Can you work these out from the model? Positions are in its coordinate system, mm. Face numbers are marked on the shaded views. A direction names the side the tool comes from. Give positions to 0.01 mm unless a question says otherwise; leave off trailing zeros. Loops run counter-clockwise (first coordinate to the right, second up) from the corner with the lowest first, then second, coordinate; pieces in that order, holes last. Notation, with made-up numbers: (-20, -38.5) - (8, -38.5) arc R6 ccw to (8, -30.5) - close; hole circle Ø6 at (79, -5.5). An arc over 180 degrees is marked (long way). Answer as a JSON object with one key per item and string values. Group by question number.
Item 1: Suppose I cut it at B-B on z = 10.25. Write out the boundary of the cut face in (x, y), and give its area (3 significant figures).
Item 2: Please list where these lines run through material, in increasing order: L1, parallel to Y at x = 7.75, z = 4.25; L2, parallel to X at y = 12.25, z = 8.25; L3, parallel to Y at x = 2, z = 1.25.
Item 3: Which directions (+Z, -Z, +X, -X, +Y, -Y) give clear straight access to the entire face, cutting with the end or side of a thin tool? Please do the marked faces 1, 2, 3, 4 and 5.
Item 4: Suppose I cut it at C-C on y = 14.5. Write out the boundary of the cut face in (x, z), and give its area (3 significant figures).
Item 5: Thinking about a two-plate mould opening in Y: for the marked faces 6, 7, 8 and 9, which applies, pulls with the +Y half, pulls with the -Y half, needs draft (parallel to the pull), parting line crosses it, or undercut?
Item 6: Will these pins go through, and if not, where does the flat tip stop? pin 1 (5 mm diameter, centred on x = 1.5, z = 6, fed in from -Y); pin 2 (3 mm diameter, centred on y = 10, z = 7, fed in from -X) (3 decimals); pin 3 (6 mm diameter, centred on x = 1, z = 3.5, fed in from -Y).
Item 7: Suppose I cut it at D-D on x = -9.5. Write out the boundary of the cut face in (y, z).
Item 8: Suppose I cut it at A-A on z = 4.25. Write out the boundary of the cut face in (x, y).
from build123d import *

# Parameters (mm, degrees)
F1_DEPTH = 12
F3_DEPTH = 10.5
F4_R     = 3
F5_R     = 1.35
F6_DEPTH = 8


with BuildPart() as f1:
    # F0 (on Top) → F1 (new body)
    with BuildSketch(Plane.XY):
        Polygon((-7.96441, 20), (-7.96441, 0), (-3.56441, 0), (-3.56441, 15.6), (12.03559, 15.6), (12.03559, 20), align=None)
    extrude(amount=F1_DEPTH)

    # F2 (on face) → F3 (cut)
    with BuildSketch(Plane.XY.offset(12)):
        Polygon((-6.66441, 0), (-5.76441, 0), (-5.76441, 17.8), (12.03559, 17.8), (12.03559, 18.7), (-6.66441, 18.7), align=None)
        Polygon((-5.76441, 17.8), (-5.76441, 0), (-4.76441, 0), (-4.76441, 16.8), (12.03559, 16.8), (12.03559, 17.8), align=None)
    extrude(amount=-F3_DEPTH, mode=Mode.SUBTRACT)

    # F4
    f4_edges = [f1.edges().sort_by_distance(p)[0] for p in [
        (-4.76441, 16.8, 6.75),
        (-3.56441, 15.6, 6),
    ]]
    fillet(f4_edges, radius=F4_R)

    # F5 (on Top) → F6 (join)
    with BuildSketch(Plane.XY):
        with BuildLine():
            ThreePointArc((-7.96441, 20), (-9.434479, 18.498851), (-11.331965, 17.59658))
            ThreePointArc((-11.331965, 17.59658), (-9.376537, 17.445554), (-7.96441, 16.084523))
            Line((-7.96441, 16.084523), (-7.96441, 20))
        make_face()
        with BuildLine():
            ThreePointArc((-7.96441, 13.515477), (-9.376537, 12.154446), (-11.331965, 12.00342))
            ThreePointArc((-11.331965, 12.00342), (-9.434479, 11.101149), (-7.96441, 9.6))
            Line((-7.96441, 9.6), (-7.96441, 13.515477))
        make_face()
        with BuildLine():
            ThreePointArc((-7.96441, 16.084523), (-9.376537, 17.445554), (-11.331965, 17.59658))
            ThreePointArc((-11.331965, 17.59658), (-13.46441, 14.8), (-11.331965, 12.00342))
            ThreePointArc((-11.331965, 12.00342), (-9.376537, 12.154446), (-7.96441, 13.515477))
            Line((-7.96441, 13.515477), (-7.96441, 16.084523))
        make_face()
        with Locations((-10.56441, 14.8)):
            Circle(F5_R, mode=Mode.SUBTRACT)
    extrude(amount=F6_DEPTH)


solid = f1.part
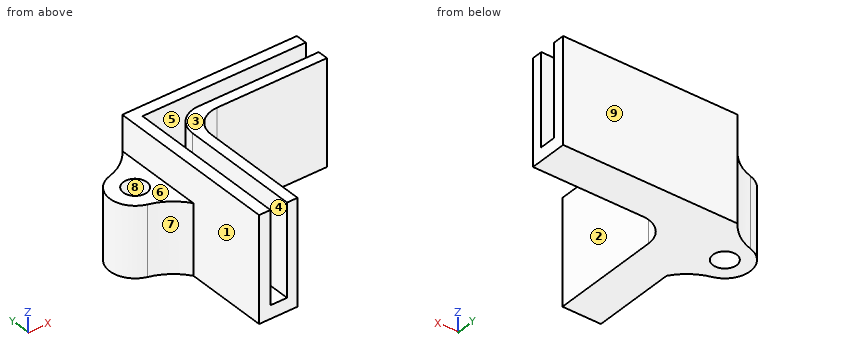
Worked out:
{
 "1": {"outline": "(-7.96, 0) - (-6.66, 0) - (-6.66, 18.7) - (12.04, 18.7) - (12.04, 20) - (-7.96, 20) - close; (-4.76, 0) - (-3.56, 0) - (-3.56, 12.6) arc R3 cw to (-0.56, 15.6) - (12.04, 15.6) - (12.04, 16.8) - (-1.76, 16.8) arc R3 ccw to (-4.76, 13.8) - close", "area": "89.2 mm2"},
 "2": {"L1": "y = 15.6 to 16.8, 18.7 to 20", "L2": "x = -7.96 to -6.66, -4.76 to -3.56", "L3": "y = 15.6 to 20"},
 "3": {"face 1": "+Z, -X, -Y", "face 2": "+Z, -Z, +X, -Y", "face 3": "+Z, +X, -X, +Y, -Y", "face 4": "+Z, -Y", "face 5": "+Z, +X"},
 "4": {"outline": "(-13.45, 0) - (-11.88, 0) - (-11.88, 8) - (-13.45, 8) - close; (-9.25, 0) - (-2.89, 0) - (-2.89, 12) - (-4.68, 12) - (-4.68, 1.5) - (-6.66, 1.5) - (-6.66, 12) - (-7.96, 12) - (-7.96, 8) - (-9.25, 8) - close", "area": "62.9 mm2"},
 "5": {"face 6": "needs draft", "face 7": "pulls with the -Y half", "face 8": "undercut", "face 9": "pulls with the +Y half"},
 "6": {"pin 1": "stops at y = 15.57", "pin 2": "stops at x = -10.075", "pin 3": "stops at y = 15.23"},
 "7": {"outline": "(11.15, 0) - (13.97, 0) - (13.97, 8) - (11.15, 8) - close; (15.63, 0) - (18.45, 0) - (18.45, 8) - (15.63, 8) - close"},
 "8": {"outline": "(-11.33, 12) arc R6 cw to (-7.96, 9.6) - (-7.96, 0) - (-6.66, 0) - (-6.66, 18.7) - (12.04, 18.7) - (12.04, 20) - (-7.96, 20) arc R6 cw to (-11.33, 17.6) arc R2.9 ccw to start; (-4.76, 0) - (-3.56, 0) - (-3.56, 12.6) arc R3 cw to (-0.56, 15.6) - (12.04, 15.6) - (12.04, 16.8) - (-1.76, 16.8) arc R3 ccw to (-4.76, 13.8) - close; hole circle Ø2.7 at (-10.56, 14.8)"}
}
